Check sheet for the modelled part. Datum: model origin and axes. Units: mm. Face numbers are marked on the shaded views. A direction names the side the tool comes from. Round coordinates to 2 decimals unless told otherwise and drop trailing zeros. Write each loop counter-clockwise with the first axis right and the second up, starting at its lowest first coordinate (ties: lowest second). Pieces come first, ordered by that corner, then holes.
Item 1: Cross-section at A-A on x = 0. Enter the section's corners in (y, z) (3 decimals), plus the area to 3 significant figures.
Item 2: Cross-section at D-D on z = 11. Enter the section's corners in (x, y).
Item 3: Cross-section at B-B on z = -5.5. Enter the section's corners in (x, y).
Item 4: Tool access check on the marked faces 5, 6, 7 and 8. Record the directions out of +Z, -Z, +X, -X, +Y, -Y that give a thin tool (end or side, any length) a straight path to the whole face; none if there is none.
Item 5: Cross-section at C-C on y = -60.5. Enter the section's corners in (x, z) (3 decimals).
Item 6: Release check for a two-part mould opening along Y. For the marked faces 1, 2, 3 and 4 record: +Y half, -Y half, draft (parallel to the pull), parting line (faces both ways), or undercut.
Item 7: Material ranges on line 1 (Z direction, x = 0, y = -42); line 2 (Y direction, x = 22.5, z = 5); line 3 (Z direction, x = 0.5, y = -8.5), recorded low to high.
Item 8: Go/stop test with flat-tipped pins: pin 1 Ø7.5 at (y, z) = (-3.5, 42.5) entering from -X; pin 2 Ø10 at (x, y) = (17, -59.5) entering from +Z (3 decimals); pin 3 Ø6 at (y, z) = (-31.5, -4) entering from -X. Record where each tip stops, or that it passes through.
from build123d import *

# Parameters (mm, degrees)
F0_R      = 25.4
F0_R_2    = 12.7
F1_DEPTH  = 76.2
F2_W      = 12.7
F2_H      = 9.525
F2_H_2    = 15.875
F3_DEPTH  = 558.8
F4_W      = 12.7
F4_H      = 9.525
F4_H_2    = 15.875
F5_DEPTH  = 279.4
F7_DEPTH  = 25.4
F9_DEPTH  = 12.7
F10_W     = 25.4
F10_H     = 12.7
F11_DEPTH = 25.4


with BuildPart() as f1:
    # F0 (on Front) → F1 (new body)
    with BuildSketch(Plane.XZ):
        Circle(F0_R)
        Circle(F0_R_2, mode=Mode.SUBTRACT)
    extrude(amount=F1_DEPTH)

    # F2 (on Right) → F3 (cut)
    with BuildSketch(Plane.YZ):
        with Locations((-57.15, -4.7625)):
            Rectangle(F2_W, F2_H)
        Polygon((-63.5, 0), (-50.8, 0), (-50.8, 25.4), (-63.5, 25.4), (-63.5, 9.525), align=None)
        with Locations((-69.85, 17.4625)):
            Rectangle(F2_W, F2_H_2)
    extrude(amount=F3_DEPTH, mode=Mode.SUBTRACT)

    # F4 (on Right) → F5 (cut)
    with BuildSketch(Plane.YZ):
        with Locations((-57.15, -4.7625)):
            Rectangle(F4_W, F4_H)
        Polygon((-63.5, 0), (-50.8, 0), (-50.8, 25.4), (-63.5, 25.4), (-63.5, 9.525), align=None)
        with Locations((-69.85, 17.4625)):
            Rectangle(F4_W, F4_H_2)
    extrude(amount=-F5_DEPTH, mode=Mode.SUBTRACT)

    # F6 (on Right) → F7 (join)
    with BuildSketch(Plane.YZ):
        Polygon((-38.1, 0), (0, 0), (0, 50.8), align=None)
    extrude(amount=F7_DEPTH)

    # F8 (on Right) → F9 (join)
    with BuildSketch(Plane.YZ):
        Polygon((-38.1, 0), (0, 0), (0, 50.8), align=None)
    extrude(amount=-F9_DEPTH)

    # F10 (on face) → F11 (cut)
    with BuildSketch(Plane(origin=(0, 0, 0), x_dir=(-1, 0, 0), z_dir=(0, 1, 0))):
        with Locations((0, 44.45)):
            Rectangle(F10_W, F10_H)
    extrude(amount=-F11_DEPTH, mode=Mode.SUBTRACT)


solid = f1.part
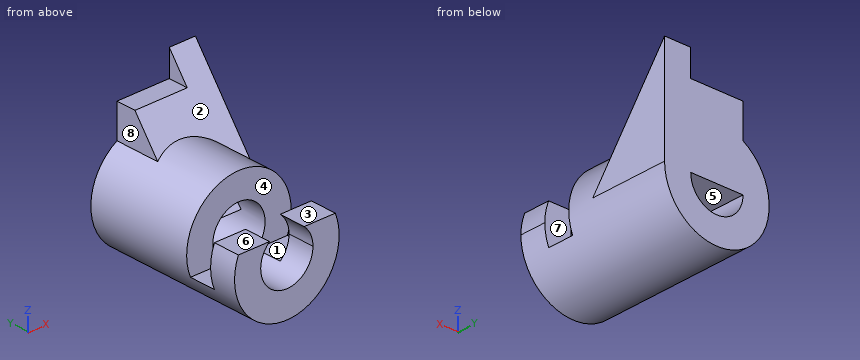
Response values:
1. outline: (-76.2, -25.4) - (0, -25.4) - (0, -12.7) - (-76.2, -12.7) - close; (-50.8, 12.7) - (-28.575, 12.7) - (-38.1, 0) - (0, 0) - (0, 38.1) - (-9.525, 38.1) - (-19.05, 25.4) - (-50.8, 25.4) - close
1. area: 2,220 mm2
2. outline: (-22.89, -50.8) - (-6.35, -50.8) - (-6.35, -29.85) - (6.35, -29.85) - (6.35, -50.8) - (22.89, -50.8) - (22.89, -29.85) - (25.4, -29.85) - (25.4, 0) - (-22.89, 0) - close
3. outline: (-24.8, -76.2) - (-11.45, -76.2) - (-11.45, -63.5) - (-24.8, -63.5) - close; (-24.8, -50.8) - (-11.45, -50.8) - (-11.45, 0) - (-24.8, 0) - close; (11.45, -76.2) - (24.8, -76.2) - (24.8, -63.5) - (11.45, -63.5) - close; (11.45, -50.8) - (24.8, -50.8) - (24.8, 0) - (11.45, 0) - close
4. face 5: +Y, -Y
4. face 6: +Z, +X, -X, -Y
4. face 7: +Z, +X, -X
4. face 8: +Z, -X, +Y, -Y
5. outline: (-23.546, -9.525) arc R25.4 ccw to (23.546, -9.525) - (8.4, -9.525) arc R12.7 cw to (-8.4, -9.525) - close
6. face 1: undercut
6. face 2: -Y half
6. face 3: draft
6. face 4: undercut
7. line 1: z = -25.4 to -12.7, 12.7 to 25.4
7. line 2: y = -76.2 to -63.5, -50.8 to 0
7. line 3: z = -25.4 to -12.69, 0 to 38.1
8. pin 1: stops at x = 12.7
8. pin 2: stops at z = 9.525
8. pin 3: stops at x = -25.38
